For this review, take the finished solid that the model builds, in its own axes (mm). A direction names the side the tool comes from. Round coordinates to 2 decimals unless told otherwise and drop trailing zeros. Order: outer loops, then holes, each group sorted by start corner. A loop starts at its lowest first (then second) coordinate and runs counter-clockwise, first axis right, second up. Notation, with made-up numbers: (-36.75, 2) -> (2.25, 2) arc R31 cw to (2.25, 27) -> close; hole circle Ø1 at (71.25, 46). An arc over 180 degrees is marked (long way). Answer in a Markdown table with one row per item.
```python
from build123d import *

# Parameters (mm, degrees)
SKETCH1_W           = 10.16
SKETCH1_H           = 5.08
BOSS_EXTRUDE1_DEPTH = 2.54
EXTRUDE_THIN1_DEPTH = 5.08


with BuildPart() as part:
    # Sketch1 → Boss-Extrude1 (new body)
    with BuildSketch(Plane(origin=(0, 0, 0), x_dir=(1, 0, 0), z_dir=(0, 1, 0))):
        with Locations((5.08, 2.54)):
            Rectangle(SKETCH1_W, SKETCH1_H)
    extrude(amount=BOSS_EXTRUDE1_DEPTH)

    # Sketch4 → Extrude-Thin1 (add)
    with BuildSketch(Plane(origin=(0, 0, 0), x_dir=(-1, 0, 0), z_dir=(0, 0, -1))):
        with BuildLine():
            ThreePointArc((-7.62, 2.54), (-2.949354511, 22.528719629), (10.095343756, 38.378000016))
            Line((10.095343756, 38.378000016), (13.180251735, 34.341944669))
            ThreePointArc((13.180251735, 34.341944669), (1.604640029, 20.277601299), (-2.54, 2.54))
            Line((-2.54, 2.54), (-7.62, 2.54))
        make_face()
    extrude(amount=EXTRUDE_THIN1_DEPTH)


solid = part.part
```
Q1. Tool access review of faces 5 (the face through (0, 1, -3)), 6 (the face through (-11.616, 36.388, -2.504)): name each direction out of +Z, -Z, +X, -X, +Y, -Y from which nothing blocks a thin tool from reaching the whole face with its end or side.
Answer key:
| item | result |
|---|---|
| face 5 | +Z, -Z, -X, -Y |
| face 6 | +Z, -Z, -X, +Y |
Q2. Take a section at D-D, the plane x = 8.75. Write out the cut boundary in (y, z), then the cut area to 3 significant figures.
Answer key:
| item | result |
|---|---|
| outline | (0, -5.08) -> (2.54, -5.08) -> (2.54, 0) -> (0, 0) -> close |
| area | 12.9 mm^2 |
Q3. Take a section at B-B, the plane z = -4.2. Write out the cut boundary in (x, y), then the cut area to 3 significant figures.
Answer key:
| item | result |
|---|---|
| outline | (-13.18, 34.34) arc R40.03 cw to (2.54, 2.54) -> (0, 2.54) -> (0, 0) -> (10.16, 0) -> (10.16, 2.54) -> (7.62, 2.54) arc R45.11 ccw to (-10.1, 38.38) -> close |
| area | 224 mm^2 |
Q4. The part is to be moulded in two halves that separate along Y. For faces 1 (the face through (5, 0, -3)), 2 (the face through (-1.72, 20.51, -2.5)), 3 (the face through (9, 2.54, -3)), 4 (the face through (1, 2.54, -3)), say which applies: +Y half, -Y half, draft (parallel to the pull), parting line (faces both ways), or undercut.
Answer key:
| item | result |
|---|---|
| face 1 | -Y half |
| face 2 | undercut |
| face 3 | +Y half |
| face 4 | undercut |
Q5. Clearance check with flat-ended pins moving along their axes: pin 1 Ø6 at (x, y) = (0.5, 22.5) entering from +Z; pin 2 Ø3 at (y, z) = (6.5, -2.5) entering from -X; pin 3 Ø0.8 at (y, z) = (0.5, -2.5) entering from -X; pin 4 Ø3 at (x, z) = (2, -2) entering from +Y. State where each tip first meets the part, or that it passes through.
Answer key:
| item | result |
|---|---|
| pin 1 | stops at z = 0 |
| pin 2 | stops at x = 2.17 |
| pin 3 | stops at x = 0 |
| pin 4 | stops at y = 26.86 |
Q6. Take a section at A-A, the plane x = 0.75. Write out the cut boundary in (y, z), then the cut area to 3 significant figures.
Answer key:
| item | result |
|---|---|
| outline | (0, -5.08) -> (2.54, -5.08) -> (2.54, 0) -> (0, 0) -> close; (14.38, -5.08) -> (26.47, -5.08) -> (26.47, 0) -> (14.38, 0) -> close |
| area | 74.3 mm^2 |
Q7. To check wall thickness, follow probe 1 along Y at (x, z) = (-2.25, -0.9); probe 2 along Y at (x, z) = (-4.5, -2.4); probe 3 along X at (y, z) = (28, -4.4). State the ranges of each line that lie inside material, in increasing order.
Answer key:
| item | result |
|---|---|
| probe 1 | y = 21.53 to 30.7 |
| probe 2 | y = 25.21 to 33.31 |
| probe 3 | x = -6.6 to -0.25 |
Q8. Take a section at C-C, the plane y = 3. Write out the cut boundary in (x, z).
Answer key:
| item | result |
|---|---|
| outline | (2.54, -5.08) -> (7.62, -5.08) -> (7.62, 0) -> (2.54, 0) -> close |
